Design review of the part built by this model. Coordinates are the model's own, in mm. A direction names the side the tool comes from. Give positions to 0.01 mm unless a question says otherwise; leave off trailing zeros. Order: outer loops, then holes, each group sorted by start corner. A loop starts at its lowest first (then second) coordinate and runs counter-clockwise, first axis right, second up.
```python
from build123d import *

# Parameters (mm, degrees)
SKETCH_1_W             = 106
SKETCH_1_H             = 60
ARDUINO_DEPTH          = 45
ARDUINO_2_DEPTH        = 102
SKETCH_3_W             = 28
SKETCH_3_H             = 6
ARDUINO_3_DEPTH        = 2
SKETCH_4_W             = 40
SKETCH_4_H             = 12
ARDUINO_4_DEPTH        = 60
ARDUINO_5_DEPTH        = 5
SKETCH_11_W            = 12
SKETCH_11_H            = 17
SKETCH_13_R            = 12.26
CUT_EXTRUDE_2679_DEPTH = 110.42948373
SKETCH_25_W            = 90
SKETCH_25_H            = 5
EXTRUDE_3075_DEPTH     = 30
EXTRUDE_3668_DEPTH     = 22
CUT_EXTRUDE_1_REACH    = 115.751
CUT_EXTRUDE_2_DEPTH    = 17.5
SKETCH_28_W            = 4.8
SKETCH_28_H            = 11.5
SKETCH_28_R            = 1.5
EXTRUDE_4845_DEPTH     = 2
FILLET_1_R             = 1
SKETCH_30_W            = 10
SKETCH_30_H            = 5
CUT_EXTRUDE_2_2_DEPTH  = 48
SKETCH_32_W            = 86.504453115
SKETCH_32_H            = 5.850542723
SKETCH_32_H_2          = 5.850542722
CUT_EXTRUDE_4_DEPTH    = 20


with BuildPart() as part:
    # 草图1 → arduino (new body)
    with BuildSketch(Plane(origin=(0, 0, 0), x_dir=(1, 0, 0), z_dir=(0, 1, 0))):
        with Locations((7.944608655, 0.410719743)):
            Rectangle(SKETCH_1_W, SKETCH_1_H)
    extrude(amount=ARDUINO_DEPTH)

    # 草图2 → arduino 2 (cut)
    with BuildSketch(Plane(origin=(60.944608655, 0, 0), x_dir=(0, 0, -1), z_dir=(1, 0, 0))):
        Polygon((-27.589280257, 22), (28.410719743, 22), (28.410719743, 2), (0.410719743, 2), (-27.589280257, 2), align=None)
    extrude(amount=-ARDUINO_2_DEPTH, mode=Mode.SUBTRACT)

    # 草图3 → arduino 3 (add)
    with BuildSketch(Plane(origin=(60.944608655, 0, 0), x_dir=(0, 0, -1), z_dir=(1, 0, 0))):
        with Locations((14.410719743, 5)):
            Rectangle(SKETCH_3_W, SKETCH_3_H)
        with Locations((-13.589280257, 5)):
            Rectangle(SKETCH_3_W, SKETCH_3_H)
    extrude(amount=-ARDUINO_3_DEPTH)

    # 草图4 → arduino 4 (cut)
    with BuildSketch(Plane(origin=(0, 0, -30.410719743), x_dir=(-1, 0, 0), z_dir=(0, 0, -1))):
        with Locations((10.055391345, 15)):
            Rectangle(SKETCH_4_W, SKETCH_4_H)
        with Locations((-29.944608655, 15)):
            Rectangle(SKETCH_4_W, SKETCH_4_H)
    extrude(amount=-ARDUINO_4_DEPTH, mode=Mode.SUBTRACT)

    # 草图7 → arduino 5 (cut)
    with BuildSketch(Plane.ZY.offset(45.055391345)):
        Polygon((-0.410719743, 22), (-28.410719743, 22), (-28.410719743, 8), (27.589280257, 8), (27.589280257, 22), align=None)
    extrude(amount=-ARDUINO_5_DEPTH, mode=Mode.SUBTRACT)

    # 草图11 → Cut-Revolve 2344 (revolve, cut)
    with BuildSketch(Plane.XY):
        with Locations((54.944608655, 31.5)):
            Rectangle(SKETCH_11_W, SKETCH_11_H)
    revolve(axis=Axis((60.944608655, 40, 0), (-1, 0, 0)), mode=Mode.SUBTRACT)

    # 草图12 → Cut-Revolve 2556 (revolve, cut)
    with BuildSketch(Plane.XY):
        Polygon((48.944608655, 25.3), (48.944608655, 40), (-34.055391345, 40), (-34.055391345, 25), align=None)
    revolve(axis=Axis((48.944608655, 40, 0), (-1, 0, 0)), mode=Mode.SUBTRACT)

    # 草图13 → Cut-Extrude 2679 (cut, through all)
    with BuildSketch(Plane(origin=(-34.055391345, 0, 0), x_dir=(0, 0, -1), z_dir=(1, 0, 0))):
        with Locations((0.410719743, 40)):
            Circle(SKETCH_13_R)
    extrude(amount=-CUT_EXTRUDE_2679_DEPTH, mode=Mode.SUBTRACT)

    # 草图25 → Extrude 3075 (add)
    with BuildSketch(Plane(origin=(0, 45, 0), x_dir=(1, 0, 0), z_dir=(0, 1, 0))):
        with Locations((15.944608655, -27.089280257)):
            Rectangle(SKETCH_25_W, SKETCH_25_H)
    extrude_3075 = extrude(amount=EXTRUDE_3075_DEPTH)

    # 草图26 → Extrude 3668 (add)
    with BuildSketch(Plane.XY.offset(29.589280257)):
        Polygon((10.244608655, 61), (10.244608655, 75), (8.244608655, 75), (8.244608655, 63.5), (-24.055391345, 63.5), (-24.055391345, 75), (-26.055391345, 75), (-26.055391345, 61), align=None)
        Polygon((8.244608655, 63.5), (8.244608655, 75), (-16.055391345, 75), (-24.055391345, 75), (-24.055391345, 63.5), align=None)
    extrude_3668 = extrude(amount=EXTRUDE_3668_DEPTH)

    # 草图26<3> → 舵机舱切除1 (cut, up to next)
    with BuildSketch(Plane.XY.offset(29.589280257), mode=Mode.PRIVATE) as cut_extrude_1_sk1:
        Polygon((8.244608655, 63.5), (8.244608655, 75), (-16.055391345, 75), (-24.055391345, 75), (-24.055391345, 63.5), align=None)
    cut_extrude_1_tool1 = extrude(cut_extrude_1_sk1.sketch, amount=-CUT_EXTRUDE_1_REACH, mode=Mode.PRIVATE) & part.part
    cut_extrude_1 = cut_extrude_1_tool1.solids().sort_by_distance((-7.905391, 69.25, 29.58928))[0]
    add(cut_extrude_1, mode=Mode.SUBTRACT)

    # 草图26<4> → Cut-Extrude 2 (cut)
    with BuildSketch(Plane.XY.offset(29.589280257)):
        Polygon((8.244608655, 63.5), (8.244608655, 75), (-16.055391345, 75), (-24.055391345, 75), (-24.055391345, 63.5), align=None)
    cut_extrude_2 = extrude(amount=CUT_EXTRUDE_2_DEPTH, mode=Mode.SUBTRACT)

    # 草图28 → Extrude 4845 (add)
    # profile 1 of 2: a face of its own
    with BuildSketch(Plane(origin=(0, 0, 24.589280257), x_dir=(-1, 0, 0), z_dir=(0, 0, -1))):
        with Locations((-5.844608655, 69.25)):
            Rectangle(SKETCH_28_W, SKETCH_28_H)
        with Locations((-5.844608655, 69.25)):
            Circle(SKETCH_28_R, mode=Mode.SUBTRACT)
    # profile 2 of 2: a face of its own
    with BuildSketch(Plane(origin=(0, 0, 24.589280257), x_dir=(-1, 0, 0), z_dir=(0, 0, -1))):
        with Locations((21.655391345, 69.25)):
            Rectangle(SKETCH_28_W, SKETCH_28_H)
        with Locations((21.655391345, 69.25)):
            Circle(SKETCH_28_R, mode=Mode.SUBTRACT)
    extrude_4845 = extrude(amount=-EXTRUDE_4845_DEPTH)

    # Mirror 4928: Extrude 3075, Extrude 3668, 舵机舱切除1, Cut-Extrude 2, Extrude 4845 across plane
    add(extrude_3075.mirror(Plane(origin=(0, 0, -0.410719743), x_dir=(1, 0, 0), z_dir=(0, 0, -1))))
    add(extrude_3668.mirror(Plane(origin=(0, 0, -0.410719743), x_dir=(1, 0, 0), z_dir=(0, 0, -1))))
    add(cut_extrude_1.mirror(Plane(origin=(0, 0, -0.410719743), x_dir=(1, 0, 0), z_dir=(0, 0, -1))), mode=Mode.SUBTRACT)
    add(cut_extrude_2.mirror(Plane(origin=(0, 0, -0.410719743), x_dir=(1, 0, 0), z_dir=(0, 0, -1))), mode=Mode.SUBTRACT)
    add(extrude_4845.mirror(Plane(origin=(0, 0, -0.410719743), x_dir=(1, 0, 0), z_dir=(0, 0, -1))))

    # 变化圆角1
    fillet_1_edges = [part.edges().sort_by_distance(p)[0] for p in [
        (-45.055391345, 45, 20.18632412),
        (-29.055391345, 60, 24.589280257),
        (-29.055391345, 60, 29.589280257),
        (-29.055391345, 75, 27.089280257),
        (10.244608655, 75, 40.589280257),
        (-26.055391345, 75, 40.589280257),
        (10.244608655, 68, 51.589280257),
        (-7.905391345, 75, 51.589280257),
        (-26.055391345, 68, 51.589280257),
        (-7.905391345, 61, 51.589280257),
        (60.944608655, 22, -0.410719743),
        (-37.055391345, 45, -30.410719743),
        (-29.055391345, 75, -27.910719743),
        (-29.055391345, 60, -30.410719743),
        (-29.055391345, 60, -25.410719743),
        (-7.905391345, 75, -52.410719743),
        (-26.055391345, 75, -41.410719743),
        (10.244608655, 75, -41.410719743),
        (-7.905391345, 61, -52.410719743),
        (-26.055391345, 68, -52.410719743),
        (-26.055391345, 61, -41.410719743),
        (10.244608655, 68, -52.410719743),
        (60.944608655, 15, 27.589280257),
        (60.944608655, 15, -28.410719743),
        (60.944608655, 8, -0.410719743),
        (-45.055391345, 45, -21.007763606),
        (-30.055391345, 15, -30.410719743),
        (9.944608655, 9, -30.410719743),
        (49.944608655, 15, 27.589280257),
        (9.944608655, 21, 29.589280257),
        (49.944608655, 15, 29.589280257),
        (-30.055391345, 15, 29.589280257),
        (9.944608655, 9, 29.589280257),
        (9.944608655, 21, -30.410719743),
        (49.944608655, 15, -30.410719743),
        (-45.055391345, 22.5, -30.410719743),
        (-45.055391345, 22.5, 29.589280257),
        (-45.055391345, 22, -0.410719743),
        (-37.055391345, 45, 29.589280257),
        (-45.055391345, 15, 27.589280257),
        (-45.055391345, 15, -28.410719743),
        (-45.055391345, 8, -0.410719743),
    ]]
    fillet(fillet_1_edges, radius=FILLET_1_R - 0.0001)  # a hair under: the kernel refuses the full size

    # 草图30 → Cut-Extrude 2 2 (cut)
    with BuildSketch(Plane(origin=(0, 75, 0), x_dir=(1, 0, 0), z_dir=(0, 1, 0))):
        with Locations((55.944608655, -27.089280257)):
            Rectangle(SKETCH_30_W, SKETCH_30_H)
        with Locations((55.944608655, 27.910719743)):
            Rectangle(SKETCH_30_W, SKETCH_30_H)
    extrude(amount=-CUT_EXTRUDE_2_2_DEPTH, mode=Mode.SUBTRACT)

    # 草图32 → 切除-拉伸4 (cut)
    with BuildSketch(Plane(origin=(0, 45, 0), x_dir=(1, 0, 0), z_dir=(0, 1, 0))):
        with Locations((3.4181604, 20.610413575)):
            Rectangle(SKETCH_32_W, SKETCH_32_H)
        with Locations((3.4181604, -19.788974089)):
            Rectangle(SKETCH_32_W, SKETCH_32_H_2)
    extrude(amount=-CUT_EXTRUDE_4_DEPTH, mode=Mode.SUBTRACT)


solid = part.part
```
1. Draft analysis for pull direction X (two halves, no side actions). For faces 1 (the face through (50.945, 51, 27)), 2 (the face through (3, 35, -17.685)), 3 (the face through (-8, 61, 40)), 4 (the face through (-8, 69, -47.911)), state which applies: pulls with the +X half, pulls with the -X half, needs draft (parallel to the pull), parting line crosses it, or undercut.
Recorded:
face 1: pulls with the +X half
face 2: undercut
face 3: needs draft
face 4: undercut
2. For pin 1 (14 mm diameter, centred on x = 16, z = -22, fed in from +Y); pin 2 (6.5 mm diameter, centred on x = -2, z = -20, fed in from +Y); pin 3 (3.5 mm diameter, centred on y = 68, z = 39, fed in from -X); pin 4 (1.5 mm diameter, centred on y = 64.5, z = -27.5, fed in from -X), all flat-tipped, find the tip position at first contact; note any pin that passes through.
Recorded:
pin 1: stops at y = 75
pin 2: stops at y = 45
pin 3: stops at x = -26.06
pin 4: stops at x = -29.06
3. Machinability: for faces 5 (the face through (48.945, 25, -1)), 6 (the face through (3, 25, -21)), 7 (the face through (-8, 61, -41)), which of the approach directions +Z, -Z, +X, -X, +Y, -Y give a long, thin tool a straight path to every point of the face, cutting with its end or side? Answer none if there is none.
Recorded:
face 5: +X
face 6: +Y
face 7: -Z, +X, -X, -Y
4. Take a section at C-C (y = 40). State how many separate pieces and enclosed holes the cut face has, then the cut area to 3 significant figures.
Recorded:
separate pieces: 2
enclosed holes: 2
area: 2,100 mm2
5. Take a section at A-A (z = -20). State the section outline as (x, y) points, then the cut area to 3 significant figures.
Recorded:
outline: (-45.06, 0) - (60.94, 0) - (60.94, 7) arc R1 ccw to (59.94, 8) - (58.94, 8) - (58.94, 2) - (-41.06, 2) - (-41.06, 8) - (-44.06, 8) arc R1 ccw to (-45.06, 7) - close; (-45.06, 23) arc R1 ccw to (-44.06, 22) - (59.94, 22) arc R1 ccw to (60.94, 23) - (60.94, 45) - (46.67, 45) - (46.67, 25) - (-39.83, 25) - (-39.83, 45) - (-44.06, 45) arc R1 ccw to (-45.06, 44) - close
area: 955 mm2
6. Take a section at B-B (y = 58.5). State the section outline as (x, z) points, then the cut area to 3 significant figures.
Recorded:
outline: (-29.06, -29.41) arc R1 ccw to (-28.06, -30.41) - (50.94, -30.41) - (50.94, -25.41) - (-28.06, -25.41) arc R1 ccw to (-29.06, -26.41) - close; (-29.06, 25.59) arc R1 ccw to (-28.06, 24.59) - (50.94, 24.59) - (50.94, 29.59) - (-28.06, 29.59) arc R1 ccw to (-29.06, 28.59) - close
area: 799 mm2
7. For line 1 along Y through (x, z) = (7.5, 9.5); line 2 along Z through (x, y) = (-23, 71); line 3 along Z through (x, y) = (-19, 39), list the stretches that pass through material, from the lowest coordinate up.
Recorded:
line 1: y = 0 to 2, 22 to 28.59
line 2: z = -52.41 to -47.91, -27.41 to -25.41, 24.59 to 26.59, 47.09 to 51.59
line 3: z = -30.41 to -23.54, -17.69 to -14.91, 14.91 to 16.86, 22.71 to 29.59
